from build123d import *

# Parameters (mm, degrees)
F0_W      = 63.5
F0_H      = 42
F0_R      = 2
F0_R_2    = 11.5
F1_DEPTH  = 4
F2_SIZE   = 4
F3_W      = 13
F3_H      = 3
F4_DEPTH  = 30
F5_R      = 5
F6_R      = 2.5
F6_R_2    = 1.75
F7_DEPTH  = 3
F8_W      = 4
F8_H      = 42
F9_DEPTH  = 22
F10_R     = 5
F11_R     = 5
F12_DEPTH = 4
F13_R     = 1.99999


# Not quite as in the source:
# - a fillet or chamfer is up to 0.001 mm smaller than in the source, because OpenCascade refuses the exact size


with BuildPart() as f1:
    # F0 (on Front) → F1 (new body)
    with BuildSketch(Plane.XZ):
        with Locations((11.25, -0.25)):
            Rectangle(F0_W, F0_H)
        with Locations((-15.25, -16)):
            Circle(F0_R, mode=Mode.SUBTRACT)
        with Locations((15.75, -16)):
            Circle(F0_R, mode=Mode.SUBTRACT)
        Circle(F0_R_2, mode=Mode.SUBTRACT)
        with Locations((-15.25, 15.5)):
            Circle(F0_R, mode=Mode.SUBTRACT)
        with Locations((15.75, 15.5)):
            Circle(F0_R, mode=Mode.SUBTRACT)
    extrude(amount=F1_DEPTH)

    # F2
    f2_edges = [f1.edges().sort_by_distance(p)[0] for p in [
        (-20.5, -2, -21.25),
        (-20.5, -2, 20.75),
    ]]
    chamfer(f2_edges, length=F2_SIZE)

    # F3 (on face) → F4 (join)
    with BuildSketch(Plane.XZ.offset(4)):
        with Locations((33.5, -5.75)):
            Rectangle(F3_W, F3_H)
    extrude(amount=F4_DEPTH)

    # F5
    f5_edges = [f1.edges().sort_by_distance(p)[0] for p in [
        (40, -34, -5.75),
        (27, -34, -5.75),
    ]]
    fillet(f5_edges, radius=F5_R)

    # F6 (on face) → F7 (cut, through all)
    with BuildSketch(Plane.XY.offset(-4.25)):
        with Locations((33.5, -21.5)):
            Circle(F6_R)
        with Locations((33.5, -30.5)):
            Circle(F6_R_2)
        with Locations((33.5, -12.5)):
            Circle(F6_R_2)
    extrude(amount=-F7_DEPTH, mode=Mode.SUBTRACT)

    # F8 (on face) → F9 (join)
    with BuildSketch(Plane.YZ.offset(43)):
        with Locations((-2, -0.25)):
            Rectangle(F8_W, F8_H)
    extrude(amount=F9_DEPTH)

    # F10
    f10_edges = [f1.edges().sort_by_distance(p)[0] for p in [
        (65, -2, -21.25),
    ]]
    fillet(f10_edges, radius=F10_R)

    # F11 (on face) → F12 (cut, through all)
    with BuildSketch(Plane.XZ.offset(4)):
        with Locations((51.7936311662, 15.85)):
            Circle(F11_R)
    extrude(amount=-F12_DEPTH, mode=Mode.SUBTRACT)

    # F13 (radius 2 in the source; OpenCascade refuses exactly that, so slightly less here)
    f13_edges = [f1.edges().sort_by_distance(p)[0] for p in [
        (51.793631, -4, 10.85),
        (51.793631, 0, 10.85),
        (50.798644, -2, 20.75),
        (52.788619, -2, 20.75),
    ]]
    fillet(f13_edges, radius=F13_R)


solid = f1.part
Here's how the part is built. I have some questions about the finished solid (model axes, mm). A direction names the side the tool comes from. Coordinates: 2 decimals unless noted, no trailing zeros. Write each loop counter-clockwise with the first axis right and the second up, starting at its lowest first coordinate (ties: lowest second). Pieces come first, ordered by that corner, then holes.
1) Thinking about a two-plate mould opening in Y: for faces 1 (the face through (33.17, -19.02, -5.73)), 2 (the face through (-18.47, -1.97, 18.78)), 3 (the face through (22, -4, -1)), 4 (the face through (22, 0, -1)), which applies, +Y half, -Y half, draft (parallel to the pull), parting line (faces both ways), or undercut?
Filled in:
face 1: undercut
face 2: draft
face 3: -Y half
face 4: +Y half
2) If we section it at A-A (x = -15.25): List the corners of the cut face in (y, z) for me, plus the area to 3 significant figures.
Filled in:
outline: (-4, -21.25) - (0, -21.25) - (0, -18) - (-4, -18) - close; (-4, -14) - (0, -14) - (0, 13.5) - (-4, 13.5) - close; (-4, 17.5) - (0, 17.5) - (0, 20.75) - (-4, 20.75) - close
area: 136 mm2
3) If we section it at D-D (x = 33.5): List the corners of the cut face in (y, z) for me.
Filled in:
outline: (-34, -7.25) - (-32.25, -7.25) - (-32.25, -4.25) - (-34, -4.25) - close; (-28.75, -7.25) - (-24, -7.25) - (-24, -4.25) - (-28.75, -4.25) - close; (-19, -7.25) - (-14.25, -7.25) - (-14.25, -4.25) - (-19, -4.25) - close; (-10.75, -7.25) - (-4, -7.25) - (-4, -21.25) - (0, -21.25) - (0, 20.75) - (-4, 20.75) - (-4, -4.25) - (-10.75, -4.25) - close
4) If we section it at C-C (x = 0): List the corners of the cut face in (y, z) for me, plus the area to 3 significant figures.
Filled in:
outline: (-4, -21.25) - (0, -21.25) - (0, -11.5) - (-4, -11.5) - close; (-4, 11.5) - (0, 11.5) - (0, 20.75) - (-4, 20.75) - close
area: 76.0 mm2
5) If I drill on line 1 (Z direction, x = 15.75, y = -0.95); line 2 (Y direction, x = 33.5, z = -6.15); line 3 (X direction, y = -1, z = 15), over which ranges is the centre line in solid material (lowest first)?
Filled in:
line 1: z = -21.25 to -18, -14 to 13.5, 17.5 to 20.75
line 2: y = -34 to -32.25, -28.75 to -24, -19 to -14.25, -10.75 to 0
line 3: x = -20.5 to -17.19, -13.31 to 13.81, 17.69 to 46.59, 56.99 to 65
6) If we section it at B-B (y = -21.5): List the corners of the cut face in (x, z) for me.
Filled in:
outline: (27, -7.25) - (31, -7.25) - (31, -4.25) - (27, -4.25) - close; (36, -7.25) - (40, -7.25) - (40, -4.25) - (36, -4.25) - close
7) Which directions (+Z, -Z, +X, -X, +Y, -Y) give clear straight access to the entire face, cutting with the end or side of a thin tool? Please do faces 5 (the face through (27, -16, -6)), 6 (the face through (63.5, -1.97, -19.82)).
Filled in:
face 5: +Z, -Z, -X, -Y
face 6: -Z, +X, +Y, -Y
8) I'm going to push flat-ended pins straight in: pin 1 (3.5 mm diameter, centred on x = 15.75, z = 15.5, fed in from +Y); pin 2 (4.5 mm diameter, centred on x = 33.5, y = -12.5, fed in from +Z); pin 3 (6.5 mm diameter, centred on x = 32.5, y = -21.5, fed in from -Z); pin 4 (3 mm diameter, centred on x = 40, z = -5.5, fed in from -Y). Where does each tip first touch, or does it pass through?
Filled in:
pin 1: passes through
pin 2: stops at z = -4.25
pin 3: stops at z = -7.25
pin 4: stops at y = -32.57
